Drawing for the job (mm, zero at the part's lowest x, y, z). A direction names the side the tool comes from. Round coordinates to 2 decimals unless told otherwise and drop trailing zeros. Order: outer loops, then holes, each group sorted by start corner. A loop starts at its lowest first (then second) coordinate and runs counter-clockwise, first axis right, second up. Notation, with made-up numbers: M 54.5,81 L 81.5,81 A20 ccw 81.5,114 Z; hole C -17.75,-13 d4. An arc over 180 degrees is marked long. One line per item, written item: value. Start each with the question number.
Item 1: Band-saw the part on B-B, the plane x = 30. Write the cut outline in (y, z), then the cut area to 3 significant figures.
Item 2: Pin check, flat tips, straight feed: pin 1 (3 mm diameter, centred on x = 15, y = 4, fed in from +Z); pin 2 (6 mm diameter, centred on y = 12.5, z = 56, fed in from +X); pin 3 (5 mm diameter, centred on y = 11.5, z = 62.5, fed in from -X); pin 4 (3 mm diameter, centred on y = 3.5, z = 45, fed in from +X). Stop position of each tip, or through.
Item 3: Band-saw the part on D-D, the plane y = 9. Write the cut outline in (x, z) (3 decimals), then the cut area to 3 significant figures.
Item 4: Band-saw the part on C-C, the plane z = 33.5. Write the cut outline in (x, y).
Item 5: Band-saw the part on A-A, the plane z = 66.31. Write the cut outline in (x, y) (3 decimals).
Item 6: Probe L1, parallel to Z at x = 15, y = 6; L2, parallel to Y at x = 2.5, z = 12; L3, parallel to Y at x = 19, z = 41.5. List the from-to ranges inside material, lowest first.
Item 7: Tool access for the marked faces 1 and 2: list every direction of +Z, -Z, +X, -X, +Y, -Y with a clear straight run to the whole face (end or side of a thin tool).
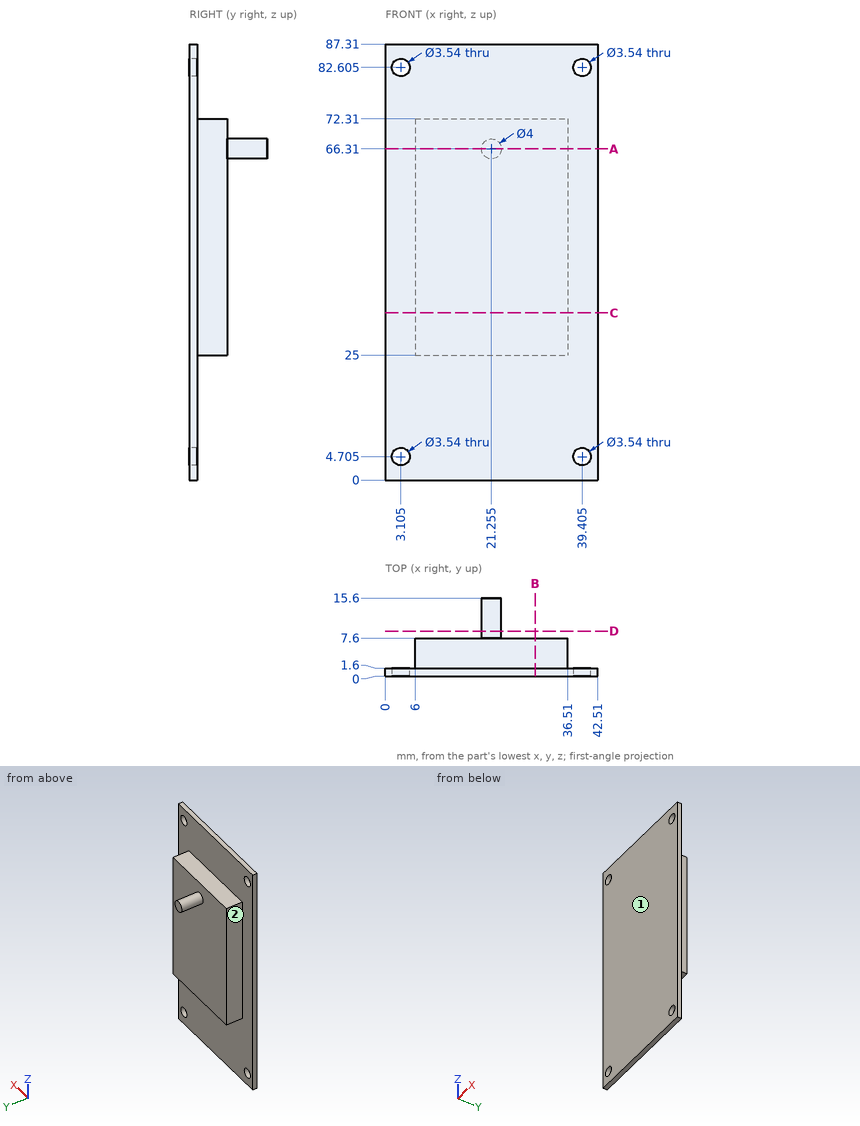
Output:
1. outline: M 0,0 L 1.6,0 L 1.6,25 L 7.6,25 L 7.6,72.31 L 1.6,72.31 L 1.6,87.31 L 0,87.31 Z
1. area: 424 mm²
2. pin 1: stops at z = 72.31
2. pin 2: passes through
2. pin 3: stops at x = 19.74
2. pin 4: stops at x = 36.51
3. outline: C 21.255,66.31 d4
3. area: 12.6 mm²
4. outline: M 0,0 L 42.51,0 L 42.51,1.6 L 36.51,1.6 L 36.51,7.6 L 6,7.6 L 6,1.6 L 0,1.6 Z
5. outline: M 0,0 L 42.51,0 L 42.51,1.6 L 36.51,1.6 L 36.51,7.6 L 23.255,7.6 L 23.255,15.6 L 19.255,15.6 L 19.255,7.6 L 6,7.6 L 6,1.6 L 0,1.6 Z
6. L1: z = 25 to 72.31
6. L2: y = 0 to 1.6
6. L3: y = 0 to 7.6
7. face 1: +Z, -Z, +X, -X, -Y
7. face 2: +Z, -Z, -X, +Y
